Build history of the part. All positions in model axes, mm. A direction names the side the tool comes from. Give positions to 0.01 mm unless a question says otherwise; leave off trailing zeros. Write each loop counter-clockwise with the first axis right and the second up, starting at its lowest first coordinate (ties: lowest second). Pieces come first, ordered by that corner, then holes.
from build123d import *

# Parameters (mm, degrees)
F1_DEPTH = 3


with BuildPart() as f1:
    # F0 (on Right) → F1 (new body)
    with BuildSketch(Plane.YZ):
        Polygon((-12.05, 42.5), (-24.1, 42.5), (-24.1, 39.5), (-32, 39.5), (-32, 31.6), (-35, 31.6), (-35, 23.7), (-32, 23.7), (-32, 15.8), (-35, 15.8), (-35, 7.9), (-32, 7.9), (-32, 0), (-32, -7.9), (-35, -7.9), (-35, -15.8), (-32, -15.8), (-32, -23.7), (-35, -23.7), (-35, -31.6), (-32, -31.6), (-32, -39.5), (-24.1, -39.5), (-24.1, -42.5), (-12.05, -42.5), (-12.05, -39.572205), (12.05, -39.572205), (12.05, -42.5), (24.1, -42.5), (24.1, -39.5), (32, -39.5), (32, -31.6), (35, -31.6), (35, -23.7), (32, -23.7), (32, -15.8), (35, -15.8), (35, -7.9), (32, -7.9), (32, 0), (32, 7.9), (35, 7.9), (35, 15.8), (32, 15.8), (32, 23.7), (35, 23.7), (35, 31.6), (32, 31.6), (32, 39.5), (24.1, 39.5), (24.1, 42.5), (12.05, 42.5), (12.05, 39.572205), (-12.05, 39.572205), align=None)
    extrude(amount=F1_DEPTH)


solid = f1.part
(1) 3-axis set-ups, long thin cutter, end or side, ignore diameter. For faces 1 (the face through (1, 28, -39.5)), 2 (the face through (1, 34, -23.7)), 3 (the face through (1, -32, 20)), 4 (the face through (1, -12.05, 41)): which of +Z, -Z, +X, -X, +Y, -Y reach the whole face in a straight line?
(2) Saw through at B-B, the plane y = -25. List the corners of the cut face in (x, z).
(3) Saw through at A-A, the plane z = 19.5. List the corners of the cut face in (x, y).
(4) Probe line 1 (Z direction, x = 2.25, y = -26); line 2 (Y direction, x = 1.7, z = -19); line 3 (Z direction, x = 2.2, y = -4.5). List the from-to ranges inside material, lowest first.
(5) Mould opens along Y. For faces 5 (the face through (1, 32, 35)), 6 (the face through (1, 33, -15.8)), 7 (the face through (1, 12.05, -41)), 8 (the face through (1, -35, -28)) say: +Y half, -Y half, draft (parallel to the pull), parting line (faces both ways), or undercut.
(6) Drop flat-ended pins along their axis: pin 1 (1.5 mm diameter, centred on x = 1, y = 33, fed in from -Z); pin 2 (1.5 mm diameter, centred on x = 1.5, y = 0, fed in from +Z); pin 3 (1.5 mm diameter, centred on x = 1, z = -41, fed in from -Y). Give the stop position or say it passes through.
Computed values:
1. face 1: -Z, +X, -X, +Y
1. face 2: +X, -X, +Y
1. face 3: +X, -X, -Y
1. face 4: +Z, +X, -X
2. outline: (0, -39.5) - (3, -39.5) - (3, 39.5) - (0, 39.5) - close
3. outline: (0, -32) - (3, -32) - (3, 32) - (0, 32) - close
4. line 1: z = -39.5 to 39.5
4. line 2: y = -32 to 32
4. line 3: z = -39.57 to 39.57
5. face 5: +Y half
5. face 6: draft
5. face 7: undercut
5. face 8: -Y half
6. pin 1: stops at z = -31.6
6. pin 2: stops at z = 39.57
6. pin 3: stops at y = -24.1
